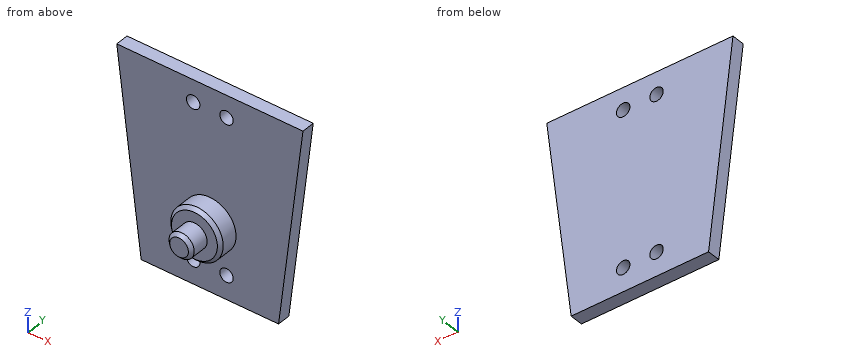
```python
from build123d import *

# Parameters (mm, degrees)
BOSS_EXTRUDE1_DEPTH            = 4
F_4_1_4_1_DIAMETER_HOLE1_D     = 4.1
F_4_1_4_1_DIAMETER_HOLE1_DEPTH = 16
CHAMFER1_SIZE                  = 1


with BuildPart() as part:
    # Sketch1 → Boss-Extrude1 (new body)
    with BuildSketch(Plane(origin=(0, -13.999999791, 0), x_dir=(1, 0, 0), z_dir=(0, 1, 0))):
        Polygon((-28.418499998, 23.757663266), (28.418499998, 23.757663266), (20.970528274, 85.000000013), (-20.970528274, 85.000000013), align=None)
    extrude(amount=-BOSS_EXTRUDE1_DEPTH)

    # Sketch2 → Revolve1 (revolve)
    with BuildSketch(Plane(origin=(0, 0, -64.665000013), x_dir=(-1, 0, 0), z_dir=(0, 0, -1)), mode=Mode.PRIVATE) as revolve1_sk:
        Polygon((-3.85, -29.999999791), (0, -29.999999791), (0, -17.999999791), (-8, -17.999999791), (-8, -23.999999791), (-3.85, -23.999999791), align=None)
    revolve(revolve1_sk.sketch.rotate(Axis((0, -29.999999791, -64.665000013), (0, 1, 0)), 180), axis=Axis((0, -29.999999791, -64.665000013), (0, 1, 0)))

    # Ø4.1 (4.1) Diameter Hole1
    with Locations(Plane(origin=(0, -13.999999791, 0), x_dir=(1, 0, 0), z_dir=(0, 1, 0))):
        with Locations((-5.085, 30.495), (5.085, 30.495), (5.085, 77.755), (-5.085, 77.755)):
            Hole(F_4_1_4_1_DIAMETER_HOLE1_D / 2, depth=F_4_1_4_1_DIAMETER_HOLE1_DEPTH)

    # Chamfer1
    chamfer1_edges = [part.edges().sort_by_distance(p)[0] for p in [
        (3.85, -29.999999791, -64.665000013),
        (8, -23.999999791, -64.665000013),
    ]]
    chamfer(chamfer1_edges, length=CHAMFER1_SIZE)


solid = part.part
```
Model file for the job. Use its own axes, mm. Round coordinates to 2 decimals unless told otherwise and drop trailing zeros. Write each loop counter-clockwise with the first axis right and the second up, starting at its lowest first coordinate (ties: lowest second). Pieces come first, ordered by that corner, then holes. Notation, with made-up numbers: (51, 21.5) - (61, 21.5) arc R32 cw to (61, 53.5) - close; hole circle Ø5 at (-26.5, 70). An arc over 180 degrees is marked (long way). Use CSV: the item, a comma, the result in double quotes. Start each with the question number.
Item 1: Band-saw the part on C-C (z = -38.5). Write the cut outline in (x, y).
Item 2: Band-saw the part on B-B (y = -16.25). State how many separate pieces and enclosed holes the cut face has, and give its area (3 significant figures).
Item 3: Band-saw the part on D-D (y = -25.25). Write the cut outline in (x, z) (3 decimals).
Item 4: Drill centre lines: L1, parallel to Y at x = -16, z = -59; L2, parallel to Z at x = 0, y = -25 (3 decimals); L3, parallel to X at y = -18.75, z = -65. Where is each one in solid material? Low to high. Write a range as [from, to].
Item 5: Pin check, flat tips, straight feed: P1, Ø2.5, axis at x = 5.085, z = -30.495, coming from the +Y side; P2, Ø6, axis at x = -16.5, z = -60, coming from the -Y side; P3, Ø5, axis at x = 5.5, z = -71.5, coming from the -Y side. Stop position of each tip, or through.
Item 6: Band-saw the part on A-A (x = 0). Write the cut outline in (y, z) (3 decimals).
Checked values:
1,outline,"(-26.63, -18) - (26.63, -18) - (26.63, -14) - (-26.63, -14) - close"
2,separate pieces,"1"
2,enclosed holes,"4"
2,area,"2,970 mm²"
3,outline,"circle Ø7.7 at (0, -64.665)"
4,L1,"y = [-18, -14]"
4,L2,"z = [-68.515, -60.815]"
4,L3,"x = [-7.99, 7.99]"
5,P1,"passes through"
5,P2,"stops at y = -18"
5,P3,"stops at y = -24"
6,outline,"(-30, -67.515) - (-29, -68.515) - (-24, -68.515) - (-24, -71.665) - (-23, -72.665) - (-18, -72.665) - (-18, -85) - (-14, -85) - (-14, -23.758) - (-18, -23.758) - (-18, -56.665) - (-23, -56.665) - (-24, -57.665) - (-24, -60.815) - (-29, -60.815) - (-30, -61.815) - close"
